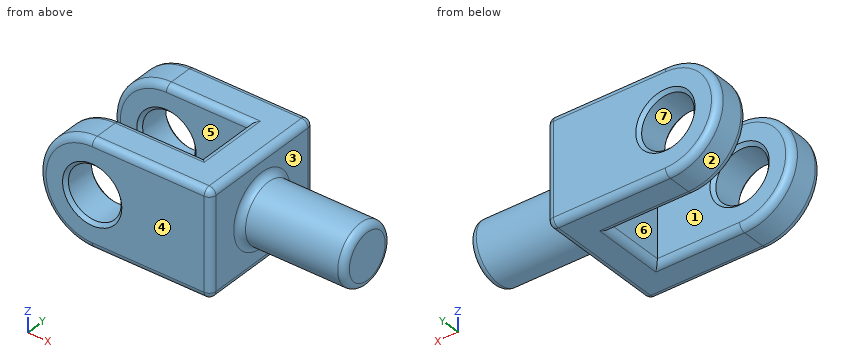
from build123d import *

# Parameters (mm, degrees)
F1_DEPTH      = 20
F1_DEPTH_BACK = 20
F2_R          = 8
F3_DEPTH      = 40.001
F4_W          = 62.5443432552
F4_H          = 18
F5_DEPTH      = 16.001
F5_DEPTH_BACK = 25
F6_R          = 9
F7_DEPTH      = 32
F8_SIZE       = 1
F9_R          = 2


with BuildPart() as f1:
    # F0 (on Front) → F1 (new body, two sides)
    with BuildSketch(Plane.XZ) as f1_sk:
        with BuildLine():
            Line((22.6247903556, -16), (22.6247903556, 16))
            Line((22.6247903556, 16), (-13.3752096444, 16))
            ThreePointArc((-13.3752096444, 16), (-29.3752096444, 0), (-13.3752096444, -16))
            Line((-13.3752096444, -16), (22.6247903556, -16))
        make_face()
    extrude(amount=F1_DEPTH)
    extrude(f1_sk.sketch, amount=-F1_DEPTH_BACK)

    # F2 (on face) → F3 (cut, through all)
    with BuildSketch(Plane.XZ.offset(20)):
        with Locations((-13.3752096444, 0)):
            Circle(F2_R)
    extrude(amount=-F3_DEPTH, mode=Mode.SUBTRACT)

    # F4 (on Top) → F5 (cut, two sides)
    with BuildSketch(Plane.XY) as f5_sk:
        with Locations((-19.647381272, 0)):
            Rectangle(F4_W, F4_H)
    extrude(amount=F5_DEPTH, mode=Mode.SUBTRACT)
    extrude(f5_sk.sketch, amount=-F5_DEPTH_BACK, mode=Mode.SUBTRACT)

    # F6 (on face) → F7 (join)
    with BuildSketch(Plane.YZ.offset(22.6247903556)):
        Circle(F6_R)
    extrude(amount=F7_DEPTH)

    # F8
    f8_edges = [f1.edges().sort_by_distance(p)[0] for p in [
        (-21.37521, -20, 0),
        (-21.37521, 20, 0),
        (-21.37521, -9, 0),
        (-21.37521, 9, 0),
    ]]
    chamfer(f8_edges, length=F8_SIZE)

    # F9
    f9_edges = [f1.edges().sort_by_distance(p)[0] for p in [
        (-29.37521, -20, 0),
        (-0.87521, -9, 16),
        (11.62479, 0, 16),
        (11.62479, 0, -16),
        (-0.87521, 9, -16),
        (-29.37521, 20, 0),
        (22.62479, 20, 0),
        (22.62479, 0, 16),
        (22.62479, -20, 0),
        (22.62479, 0, -16),
        (54.62479, -9, 0),
        (22.62479, -9, 0),
    ]]
    fillet(f9_edges, radius=F9_R)


solid = f1.part
The model under review builds one solid part; all positions refer to its coordinate system, in mm. Face numbers are marked on the shaded views. A direction names the side the tool comes from. Give positions to 0.01 mm unless a question says otherwise; leave off trailing zeros. Write each loop counter-clockwise with the first axis right and the second up, starting at its lowest first coordinate (ties: lowest second). Pieces come first, ordered by that corner, then holes. Notation, with made-up numbers: M -6.5,-10.5 L 10.5,-10.5 A26 ccw 10.5,23.5 Z; hole C 13,80 d5. An arc over 180 degrees is marked long. One line per question, with ' | ' between items. Start each with the question number.
Item 1: We need section D-D on x = 39.5. Write out the cut boundary in (y, z), plus the area to 3 significant figures.
Item 2: For pin 1 (2 mm diameter, centred on x = 6, y = -8.5, fed in from -Z); pin 2 (4 mm diameter, centred on x = -9, z = -1.5, fed in from +Y); pin 3 (9 mm diameter, centred on y = 3, z = -0.5, fed in from -X); pin 4 (10 mm diameter, centred on y = 13.5, z = -9, fed in from -X), all flat-tipped, find the tip position at first contact; note any pin that passes through.
Item 3: Draft analysis for pull direction Y (two halves, no side actions). For the marked faces 4, 5, 6 and 7, state which applies: released by +Y, released by -Y, zero draft, split by the parting line, or undercut.
Item 4: We need section A-A on z = 0. Give the number of separate pieces and of enclosed holes in the cut face, plus the area to 3 significant figures.
Item 5: Wall thickness on line 1 (Y direction, x = 3, z = 0); line 2 (X direction, y = -7.5, z = 12); line 3 (X direction, y = -14, z = -4.5): over which ranges is each line inside the solid? List them lowest first. Write a range as from..to.
Item 6: We need section B-B on y = 0. Write out the cut boundary in (x, z).
Item 7: For the marked faces 1, 2 and 3, list the 3-axis set-ups (+Z, -Z, +X, -X, +Y, -Y) from which the entire face can be reached by the end or side of a thin tool; tool diameter is ignored.
Results found:
1) outline: C 0,0 d18 | area: 254 mm2
2) pin 1: stops at z = -15.32 | pin 2: passes through | pin 3: stops at x = 11.62 | pin 4: stops at x = -28.87
3) face 4: released by -Y | face 5: undercut | face 6: undercut | face 7: zero draft
4) separate pieces: 3 | enclosed holes: 0 | area: 1,560 mm2
5) line 1: y = -20..-9, 9..20 | line 2: x = 11.62..22.62 | line 3: x = -28.73..-19.99, -6.76..22.62
6) outline: M 11.62,-14 A2 ccw 13.62,-16 L 20.62,-16 A2 ccw 22.62,-14 L 22.62,-11 A2 cw 24.62,-9 L 52.62,-9 A2 ccw 54.62,-7 L 54.62,7 A2 ccw 52.62,9 L 24.62,9 A2 cw 22.62,11 L 22.62,14 A2 ccw 20.62,16 L 13.62,16 A2 ccw 11.62,14 Z
7) face 1: +Z, -Z, -X | face 2: -X, +Y, -Y | face 3: +X
